```python
from build123d import *

# Parameters (mm, degrees)
F0_W           = 50
F0_H           = 50
F1_DEPTH       = 5
F3_D           = 5
F3_DEPTH       = 12
F3_CSINK_D     = 10
F3_CSINK_ANGLE = 60


with BuildPart() as f1:
    # F0 (on Top) → F1 (new body)
    with BuildSketch(Plane.XY):
        Rectangle(F0_W, F0_H)
    extrude(amount=F1_DEPTH)

    # F3
    with Locations(Plane.XY.offset(5)):
        with Locations((9, 15.588457), (18, 0), (9, -15.588457), (-9, -15.588457), (-18, 0), (-9, 15.588457)):
            CounterSinkHole(F3_D / 2, F3_CSINK_D / 2, depth=F3_DEPTH, counter_sink_angle=F3_CSINK_ANGLE)


solid = f1.part
```
Can you work these out from the model? Positions are in its coordinate system, mm. Coordinates: 2 decimals unless noted, no trailing zeros. Write each loop counter-clockwise with the first axis right and the second up, starting at its lowest first coordinate (ties: lowest second). Pieces come first, ordered by that corner, then holes. Notation, with made-up numbers: (6.5, 0.25) - (12.5, 0.25) arc R31 ccw to (12.5, 34.25) - close; hole circle Ø4 at (13.25, 47). An arc over 180 degrees is marked (long way). Return JSON: item names as keys, results as strings.
Q1. If we section it at D-D (z = 2.45): Please give me the cut outline in (x, y).
Computed values:
{"outline": "(-25, -25) - (25, -25) - (25, 25) - (-25, 25) - close; hole circle Ø7.06 at (-18, 0); hole circle Ø7.06 at (-9, -15.59); hole circle Ø7.06 at (-9, 15.59); hole circle Ø7.06 at (9, -15.59); hole circle Ø7.06 at (9, 15.59); hole circle Ø7.06 at (18, 0)"}
Q2. Please list where these lines run through material, in increasing order: L1, parallel to X at y = 0, z = 0.55; L2, parallel to Y at x = 9, z = 0.3; L3, parallel to Y at x = 10, z = 2.7. Write a range as from..to.
Computed values:
{"L1": "x = -25..-20.5, -15.5..15.5, 20.5..25", "L2": "y = -25..-18.09, -13.09..13.09, 18.09..25", "L3": "y = -25..-19.12, -12.06..12.06, 19.12..25"}
Q3. If we section it at A-A (x = -9): Please give me the cut outline in (y, z), then the cut area to 3 significant figures.
Computed values:
{"outline": "(-25, 0) - (-18.09, 0) - (-18.09, 0.67) - (-20.59, 5) - (-25, 5) - close; (-13.09, 0) - (13.09, 0) - (13.09, 0.67) - (10.59, 5) - (-10.59, 5) - (-13.09, 0.67) - close; (18.09, 0) - (25, 0) - (25, 5) - (20.59, 5) - (18.09, 0.67) - close", "area": "178 mm2"}
Q4. I'm going to push flat-ended pins straight in: pin 1 Ø6.5 at (x, y) = (-18, 0) entering from +Z; pin 2 Ø3 at (x, y) = (-7, -4) entering from -Z; pin 3 Ø6 at (x, y) = (9, -15.59) entering from +Z. Where does each tip first touch, or does it pass through?
Computed values:
{"pin 1": "stops at z = 1.97", "pin 2": "stops at z = 0", "pin 3": "stops at z = 1.54"}
Q5. Thinking about a two-plate mould opening in Y: for faces 1 (the flat face through (0, -25, 2)), 2 (the cylindrical face through (-8.458, 13.148, 0.33)), 3 (the flat face through (0, 0, 0)), which applies, +Y half, -Y half, draft (parallel to the pull), parting line (faces both ways), or undercut?
Computed values:
{"face 1": "-Y half", "face 2": "undercut", "face 3": "draft"}
Q6. If we section it at C-C (x = -18): Please give me the cut outline in (y, z), then the cut area to 3 significant figures.
Computed values:
{"outline": "(-25, 0) - (-2.5, 0) - (-2.5, 0.67) - (-5, 5) - (-25, 5) - close; (2.5, 0) - (25, 0) - (25, 5) - (5, 5) - (2.5, 0.67) - close", "area": "214 mm2"}
Q7. If we section it at B-B (y = 0): Please give me the cut outline in (x, z), then the cut area to 3 significant figures.
Computed values:
{"outline": "(-25, 0) - (-20.5, 0) - (-20.5, 0.67) - (-23, 5) - (-25, 5) - close; (-15.5, 0) - (15.5, 0) - (15.5, 0.67) - (13, 5) - (-13, 5) - (-15.5, 0.67) - close; (20.5, 0) - (25, 0) - (25, 5) - (23, 5) - (20.5, 0.67) - close", "area": "178 mm2"}
